Build history of the part. All positions in model axes, mm. A direction names the side the tool comes from. Give positions to 0.01 mm unless a question says otherwise; leave off trailing zeros. Order: outer loops, then holes, each group sorted by start corner. A loop starts at its lowest first (then second) coordinate and runs counter-clockwise, first axis right, second up. Notation, with made-up numbers: M -12.5,19.25 L -7.5,19.25 A22 ccw -7.5,32.25 Z; hole C -25,16 d2. An arc over 180 degrees is marked long. Answer as CSV lines item,"result".
Autodesk Inventor part; units mm, degrees
ref_plane "YZ Plane" through (0, 0, 0) normal (1, 0, 0) x (0, 1, 0)
ref_plane "XZ Plane" through (0, 0, 0) normal (0, 1, 0) x (-1, 0, 0)
ref_plane "XY Plane" through (0, 0, 0) normal (0, 0, 1) x (1, 0, 0)
sketch "Sketch1" plane through (0, 0, 0) normal (0, 1, 0) x (-1, 0, 0)
  line L0 (0, 0) -> (-18, 0)
  line L1 (-18, 0) -> (-18, -40)
  line L2 (-18, -40) -> (0, -40)
  line L3 (0, -40) -> (0, 0)
  line L4 (-1.35, 0) -> (-1.35, -40)
  line L5 (0, -1.35) -> (-18, -1.35)
  line L6 (0, -38.65) -> (-18, -38.65)
  circle A0 centre (-2.85, -2.85) radius 1.5
  circle A1 centre (-2.85, -37.15) radius 1.5
  line L7 (-8.1, -21.2) -> (-14.6, -21.2)
  line L8 (-14.6, -21.2) -> (-14.6, -31.7)
  line L9 (-14.6, -31.7) -> (-8.1, -31.7)
  line L10 (-8.1, -31.7) -> (-8.1, -21.2)
  line L11 (-6, -1) -> (-17, -1)
  line L12 (-17, -1) -> (-17, -14)
  line L13 (-17, -14) -> (-6, -14)
  line L14 (-6, -14) -> (-6, -1)
  point P0 (-6, -1.35)
  point P1 (-17, -1.35)
  dimension "d0" = 18
  dimension "d1" = 40
  dimension "d2" = 1.35
  dimension "d3" = 1.35
  dimension "d4" = 1.35
  dimension "d5" = 3
  dimension "d6" = 3
  dimension "d7" = 6.5
  dimension "d8" = 10.5
  dimension "d11" = 8.1
  dimension "d12" = 8.3
  dimension "d13" = 11
  dimension "d14" = 13
  dimension "d16" = 1
  dimension "d17" = 1
extrude "Extrusion1" add sketch "Sketch1" against normal blind 0.8 contours L3 L5 L4 L0 | L4 L5 L14 L11 L12 L1 L0 | L3 L6 L4 L5 | L4 A0 L5 | L3 L2 L4 L6 | L5 L12 L13 L14 A0 L4 A1 L6 L1 | L6 A1 L4 | L4 L2 L1 L6 | L12 L11 L14 L5 | L5 L14 L13 L12 | L10 L9 L8 L7
extrude "Extrusion2" add sketch "Sketch1" along normal blind 4.5 contours L5 L14 L13 L12
extrude "Extrusion3" add sketch "Sketch1" along normal blind 4.5 contours L10 L9 L8 L7
chamfer "Chamfer1" distance 2 angle 45 2 edges at (8.1, 0, -26.45) (14.6, 0, -26.45)
properties part number "interface_board"
Item 1: Probe line 1 along Z through (x, y) = (2.85, -0.35); line 2 along X through (y, z) = (-0.5, -2.85); line 3 along Z through (x, y) = (13, 0.6). List the from-to ranges inside material, lowest first. Write a range as from..to.
Geometry says:
line 1,"z = -40..-38.65, -35.65..-4.35, -1.35..0"
line 2,"x = 0..1.35, 4.35..18"
line 3,"z = -31.7..-21.2, -14..-1.35"
Item 2: Band-saw the part on C-C (z = -2.85). Give the cut face in (x, y).
Geometry says:
outline,"M 0,-0.8 L 1.35,-0.8 L 1.35,0 L 0,0 Z; M 4.35,-0.8 L 18,-0.8 L 18,0 L 17,0 L 17,4.5 L 6,4.5 L 6,0 L 4.35,0 Z"
Item 3: Drop flat-ended pins along their axis: pin 1 (2.5 mm diameter, centred on x = 13, y = 1.5, fed in from +Z); pin 2 (3.5 mm diameter, centred on x = 2.85, z = -2.85, fed in from -Y); pin 3 (1.2 mm diameter, centred on y = 3.5, z = -25.5, fed in from +X); pin 4 (3 mm diameter, centred on y = 3, z = -25, fed in from -X). Give the stop position or say it passes through.
Geometry says:
pin 1,"stops at z = -1.35"
pin 2,"stops at y = -0.8"
pin 3,"stops at x = 14.6"
pin 4,"stops at x = 7.6"
Item 4: Band-saw the part on A-A (x = 2.85). Give the cut face in (y, z).
Geometry says:
outline,"M -0.8,-40 L 0,-40 L 0,-38.65 L -0.8,-38.65 Z; M -0.8,-35.65 L 0,-35.65 L 0,-4.35 L -0.8,-4.35 Z; M -0.8,-1.35 L 0,-1.35 L 0,0 L -0.8,0 Z"
Item 5: Pull direction Z, two halves, no side cores. Call faces 5 (the flat face through (11, 2, -21.2)), 6 (the flat face through (11, 2, -1.35)), 7 (the flat face through (11, 2, -31.7)), 8 (the flat face through (9, -0.8, -20)): released by +Z, released by -Z, zero draft, split by the parting line, or undercut.
Geometry says:
face 5,"undercut"
face 6,"released by +Z"
face 7,"released by -Z"
face 8,"zero draft"
Item 6: 3-axis set-ups, long thin cutter, end or side, ignore diameter. For faces 1 (the flat face through (15.6, 1, -26.4)), 2 (the flat face through (7.1, 1, -26.5)), 3 (the flat face through (6, 2, -8)), 4 (the flat face through (17, 2, -8)): which of +Z, -Z, +X, -X, +Y, -Y reach the whole face in a straight line?
Geometry says:
face 1,"-Z, +X, +Y"
face 2,"-Z, -X, +Y"
face 3,"+Z, -Z, -X, +Y"
face 4,"+Z, -Z, +X, +Y"
Item 7: Band-saw the part on B-B (y = 3.2). Give the cut face in (x, z), and give its area (3 significant figures).
Geometry says:
outline,"M 6,-14 L 17,-14 L 17,-1.35 L 6,-1.35 Z; M 8.1,-31.7 L 14.6,-31.7 L 14.6,-21.2 L 8.1,-21.2 Z"
area,"207 mm2"
Item 8: Band-saw the part on D-D (x = 11). Give the cut face in (y, z), and give its area (3 significant figures).
Geometry says:
outline,"M -0.8,-40 L 0,-40 L 0,-31.7 L 4.5,-31.7 L 4.5,-21.2 L 0,-21.2 L 0,-14 L 4.5,-14 L 4.5,-1.35 L 0,-1.35 L 0,0 L -0.8,0 Z"
area,"136 mm2"
